Check sheet for the modelled part. Datum: model origin and axes. Units: mm. Face numbers are marked on the shaded views. A direction names the side the tool comes from. Give positions to 0.01 mm unless a question says otherwise; leave off trailing zeros. Loops run counter-clockwise (first coordinate to the right, second up) from the corner with the lowest first, then second, coordinate; pieces in that order, holes last. Notation, with made-up numbers: M 3,60.25 L 48,60.25 A18 cw 48,75.25 Z; hole C -12.75,65.25 d3. An arc over 180 degrees is marked long. One line per question, with ' | ' between items. Start each with the question number.
from build123d import *

# Parameters (mm, degrees)
F0_W         = 25.4
F0_H         = 25.4
F0_R         = 11.45
F1_DEPTH     = 7.62
F2_T1_DEPTH  = 25.4
F2_T3_DEPTH  = 25.4
F2_T5_DEPTH  = 25.4
F2_T7_DEPTH  = 25.4
F2_T10_ANGLE = 89.4745768315
F2_T12_ANGLE = 89.4745768315
F2_T14_ANGLE = 89.4745768315
F2_T16_ANGLE = 89.4745768315
F2_T18_ANGLE = 89.4745768315
F2_T20_ANGLE = 89.4745768315
F2_T22_ANGLE = 89.4745768315
F2_T24_ANGLE = 89.4745768315
F2_T29_DEPTH = 38.4641495789
F2_T33_DEPTH = 38.4641495789
F2_T40_DEPTH = 38.4641495789
F2_T44_DEPTH = 38.4641495789
F2_T51_DEPTH = 38.4641495789
F2_T55_DEPTH = 38.4641495789
F2_T62_DEPTH = 38.4641495789
F2_T66_DEPTH = 38.4641495789


# Not quite as in the source:
# - a fillet or chamfer that OpenCascade refuses, or shapes differently, is made with other operations: its cross-section is extruded or revolved along the edge and cut away or added


with BuildPart() as f1:
    # F0 (on Top) → F1 (new body)
    with BuildSketch(Plane.XY):
        Rectangle(F0_W, F0_H)
        Circle(F0_R, mode=Mode.SUBTRACT)
        with BuildLine():
            Line((8.4598493137, -38.1), (12.7, -38.1))
            Line((12.7, -38.1), (12.7, -12.7))
            Line((12.7, -12.7), (-12.7, -12.7))
            Line((-12.7, -12.7), (-12.7, -38.1))
            Line((-12.7, -38.1), (-8.4598493137, -38.1))
            ThreePointArc((-8.4598493137, -38.1), (0, -33.3121), (8.4598493137, -38.1))
        make_face()
        with BuildLine():
            ThreePointArc((0, -60.0970452561), (9.2970452561, -50.8), (12.7, -38.1))
            Line((12.7, -38.1), (8.4598493137, -38.1))
            ThreePointArc((8.4598493137, -38.1), (9.5093742552, -40.5442360341), (9.8679, -43.18))
            ThreePointArc((9.8679, -43.18), (-2.6357639659, -52.6893742552), (-8.4598493137, -38.1))
            Line((-8.4598493137, -38.1), (-12.7, -38.1))
            ThreePointArc((-12.7, -38.1), (-9.2970452561, -50.8), (0, -60.0970452561))
        make_face()
        with BuildLine():
            Line((38.1, -8.4598493137), (38.1, -12.7))
            ThreePointArc((38.1, -12.7), (50.8, -9.2970452561), (60.0970452561, 0))
            ThreePointArc((60.0970452561, 0), (50.8, 9.2970452561), (38.1, 12.7))
            Line((38.1, 12.7), (38.1, 8.4598493137))
            ThreePointArc((38.1, 8.4598493137), (48.0403764468, 8.5879095946), (53.0479, 0))
            ThreePointArc((53.0479, 0), (48.0403764468, -8.5879095946), (38.1, -8.4598493137))
        make_face()
        with BuildLine():
            Line((12.7, 12.7), (12.7, -12.7))
            Line((12.7, -12.7), (38.1, -12.7))
            Line((38.1, -12.7), (38.1, -8.4598493137))
            ThreePointArc((38.1, -8.4598493137), (33.3121, 0), (38.1, 8.4598493137))
            Line((38.1, 8.4598493137), (38.1, 12.7))
            Line((38.1, 12.7), (12.7, 12.7))
        make_face()
        with BuildLine():
            Line((-12.7, 12.7), (12.7, 12.7))
            Line((12.7, 12.7), (12.7, 38.1))
            Line((12.7, 38.1), (8.4598493137, 38.1))
            ThreePointArc((8.4598493137, 38.1), (0, 33.3121), (-8.4598493137, 38.1))
            Line((-8.4598493137, 38.1), (-12.7, 38.1))
            Line((-12.7, 38.1), (-12.7, 12.7))
        make_face()
        with BuildLine():
            Line((8.4598493137, 38.1), (12.7, 38.1))
            ThreePointArc((12.7, 38.1), (9.2970452561, 50.8), (0, 60.0970452561))
            ThreePointArc((0, 60.0970452561), (-9.2970452561, 50.8), (-12.7, 38.1))
            Line((-12.7, 38.1), (-8.4598493137, 38.1))
            ThreePointArc((-8.4598493137, 38.1), (-2.6357639659, 52.6893742552), (9.8679, 43.18))
            ThreePointArc((9.8679, 43.18), (9.5093742552, 40.5442360341), (8.4598493137, 38.1))
        make_face()
        with BuildLine():
            ThreePointArc((-60.0970452561, 0), (-50.8, -9.2970452561), (-38.1, -12.7))
            Line((-38.1, -12.7), (-38.1, -8.4598493137))
            ThreePointArc((-38.1, -8.4598493137), (-53.0479, 0), (-38.1, 8.4598493137))
            Line((-38.1, 8.4598493137), (-38.1, 12.7))
            ThreePointArc((-38.1, 12.7), (-50.8, 9.2970452561), (-60.0970452561, 0))
        make_face()
        with BuildLine():
            Line((-38.1, -12.7), (-12.7, -12.7))
            Line((-12.7, -12.7), (-12.7, 12.7))
            Line((-12.7, 12.7), (-38.1, 12.7))
            Line((-38.1, 12.7), (-38.1, 8.4598493137))
            ThreePointArc((-38.1, 8.4598493137), (-34.5920904054, 4.8603764468), (-33.3121, 0))
            ThreePointArc((-33.3121, 0), (-34.5920904054, -4.8603764468), (-38.1, -8.4598493137))
            Line((-38.1, -8.4598493137), (-38.1, -12.7))
        make_face()
    extrude(amount=F1_DEPTH)

    # F2: chamfer of 5.08 on 8 edges, made by hand

    # F2_s2 → F2_t1 (cut)
    with BuildSketch(Plane.YZ.offset(-38.1)):
        Polygon((-12.7, 2.54), (-7.62, 7.62), (-12.7, 7.62), align=None)
        Polygon((12.7, 2.54), (7.62, 7.62), (12.7, 7.62), align=None)
    extrude(amount=F2_T1_DEPTH, mode=Mode.SUBTRACT)

    # F2_s4 → F2_t3 (cut)
    with BuildSketch(Plane.XZ.offset(12.7)):
        Polygon((-12.7, 2.54), (-7.62, 7.62), (-12.7, 7.62), align=None)
        Polygon((12.7, 2.54), (7.62, 7.62), (12.7, 7.62), align=None)
    extrude(amount=F2_T3_DEPTH, mode=Mode.SUBTRACT)

    # F2_s6 → F2_t5 (cut)
    with BuildSketch(Plane.YZ.offset(12.7)):
        Polygon((-12.7, 2.54), (-7.62, 7.62), (-12.7, 7.62), align=None)
        Polygon((12.7, 2.54), (7.62, 7.62), (12.7, 7.62), align=None)
    extrude(amount=F2_T5_DEPTH, mode=Mode.SUBTRACT)

    # F2_s8 → F2_t7 (cut)
    with BuildSketch(Plane.XZ.offset(-38.1)):
        Polygon((12.7, 2.54), (7.62, 7.62), (12.7, 7.62), align=None)
        Polygon((-12.7, 2.54), (-7.62, 7.62), (-12.7, 7.62), align=None)
    extrude(amount=F2_T7_DEPTH, mode=Mode.SUBTRACT)

    # F2_s9 → F2_t10 (revolve, cut)
    with BuildSketch(Plane.YZ.offset(-38.1)):
        Polygon((12.7, 2.54), (7.62, 7.62), (12.7, 7.62), align=None)
    revolve(axis=Axis((-38.1, -12.7, 7.62), (0, 0, 1)), revolution_arc=F2_T10_ANGLE, mode=Mode.SUBTRACT)

    # F2_s11 → F2_t12 (revolve, cut)
    with BuildSketch(Plane(origin=(13.0483033064, 0.1196610486, 0), x_dir=(0, 0, 1), z_dir=(0.9999579525, 0.0091702357, 0))):
        Polygon((2.54, -63.3819359967), (7.62, -58.3019359967), (7.62, -63.3819359967), align=None)
    revolve(axis=Axis((12.7, 38.1, 7.62), (0, 0, 1)), revolution_arc=F2_T12_ANGLE, mode=Mode.SUBTRACT)

    # F2_s13 → F2_t14 (revolve, cut)
    with BuildSketch(Plane.XZ.offset(-38.1)):
        Polygon((12.7, 2.54), (7.62, 7.62), (12.7, 7.62), align=None)
    revolve(axis=Axis((-12.7, 38.1, 7.62), (0, 0, 1)), revolution_arc=F2_T14_ANGLE, mode=Mode.SUBTRACT)

    # F2_s15 → F2_t16 (revolve, cut)
    with BuildSketch(Plane(origin=(0.1196610486, -13.0483033064, 0), x_dir=(0, 0, 1), z_dir=(0.0091702357, -0.9999579525, 0))):
        Polygon((2.54, -63.3819359967), (7.62, -58.3019359967), (7.62, -63.3819359967), align=None)
    revolve(axis=Axis((38.1, -12.7, 7.62), (0, 0, 1)), revolution_arc=F2_T16_ANGLE, mode=Mode.SUBTRACT)

    # F2_s17 → F2_t18 (revolve, cut)
    with BuildSketch(Plane.YZ.offset(38.1)):
        Polygon((-12.7, 2.54), (-7.62, 7.62), (-12.7, 7.62), align=None)
    revolve(axis=Axis((38.1, 12.7, 7.62), (0, 0, 1)), revolution_arc=F2_T18_ANGLE, mode=Mode.SUBTRACT)

    # F2_s19 → F2_t20 (revolve, cut)
    with BuildSketch(Plane(origin=(-13.0483033064, -0.1196610486, 0), x_dir=(0, 0, 1), z_dir=(-0.9999579525, -0.0091702357, 0))):
        Polygon((2.54, -63.3819359967), (7.62, -58.3019359967), (7.62, -63.3819359967), align=None)
    revolve(axis=Axis((-12.7, -38.1, 7.62), (0, 0, 1)), revolution_arc=F2_T20_ANGLE, mode=Mode.SUBTRACT)

    # F2_s21 → F2_t22 (revolve, cut)
    with BuildSketch(Plane.XZ.offset(38.1)):
        Polygon((-12.7, 2.54), (-7.62, 7.62), (-12.7, 7.62), align=None)
    revolve(axis=Axis((12.7, -38.1, 7.62), (0, 0, 1)), revolution_arc=F2_T22_ANGLE, mode=Mode.SUBTRACT)

    # F2_s23 → F2_t24 (revolve, cut)
    with BuildSketch(Plane(origin=(-0.1196610486, 13.0483033064, 0), x_dir=(0, 0, 1), z_dir=(-0.0091702357, 0.9999579525, 0))):
        Polygon((2.54, -63.3819359967), (7.62, -58.3019359967), (7.62, -63.3819359967), align=None)
    revolve(axis=Axis((-38.1, 12.7, 7.62), (0, 0, 1)), revolution_arc=F2_T24_ANGLE, mode=Mode.SUBTRACT)


with BuildPart() as f2_tool27:
    # F2_s28 → F2_t29 (new body)
    with BuildSketch(Plane.YZ.offset(-38.1)):
        Polygon((-12.7, 2.54), (-7.62, 7.62), (-12.7, 7.62), align=None)
    extrude(amount=F2_T29_DEPTH)

    split(bisect_by=Plane.YZ.offset(-12.7), keep=Keep.TOP)


with BuildPart() as f2_tool31:
    # F2_s32 → F2_t33 (new body)
    with BuildSketch(Plane.XZ.offset(-0.3641495789)):
        Polygon((-12.7, 2.54), (-7.62, 7.62), (-12.7, 7.62), align=None)
    extrude(amount=F2_T33_DEPTH)

    split(bisect_by=Plane.XZ.offset(12.7), keep=Keep.BOTTOM)


with BuildPart() as f2_tool27_1:
    add(f2_tool27.part)

    # F2_t35: intersect F2_tool31
    add(f2_tool31.part, mode=Mode.INTERSECT)


with BuildPart() as f1_1:
    add(f1.part)

    # F2_t25: cut F2_tool27
    add(f2_tool27_1.part, mode=Mode.SUBTRACT)


with BuildPart() as f2_tool38:
    # F2_s39 → F2_t40 (new body)
    with BuildSketch(Plane.XZ.offset(38.1)):
        Polygon((12.7, 2.54), (7.62, 7.62), (12.7, 7.62), align=None)
    extrude(amount=-F2_T40_DEPTH)

    split(bisect_by=Plane.XZ.offset(12.7), keep=Keep.BOTTOM)


with BuildPart() as f2_tool42:
    # F2_s43 → F2_t44 (new body)
    with BuildSketch(Plane.YZ.offset(-0.3641495789)):
        Polygon((-12.7, 2.54), (-7.62, 7.62), (-12.7, 7.62), align=None)
    extrude(amount=F2_T44_DEPTH)

    split(bisect_by=Plane.YZ.offset(12.7), keep=Keep.BOTTOM)


with BuildPart() as f2_tool38_1:
    add(f2_tool38.part)

    # F2_t46: intersect F2_tool42
    add(f2_tool42.part, mode=Mode.INTERSECT)


with BuildPart() as f1_2:
    add(f1_1.part)

    # F2_t36: cut F2_tool38
    add(f2_tool38_1.part, mode=Mode.SUBTRACT)


with BuildPart() as f2_tool49:
    # F2_s50 → F2_t51 (new body)
    with BuildSketch(Plane.YZ.offset(38.1)):
        Polygon((12.7, 2.54), (7.62, 7.62), (12.7, 7.62), align=None)
    extrude(amount=-F2_T51_DEPTH)

    split(bisect_by=Plane.YZ.offset(12.7), keep=Keep.BOTTOM)


with BuildPart() as f2_tool53:
    # F2_s54 → F2_t55 (new body)
    with BuildSketch(Plane.XZ.offset(0.3641495789)):
        Polygon((12.7, 2.54), (7.62, 7.62), (12.7, 7.62), align=None)
    extrude(amount=-F2_T55_DEPTH)

    split(bisect_by=Plane.XZ.offset(-12.7), keep=Keep.TOP)


with BuildPart() as f2_tool49_1:
    add(f2_tool49.part)

    # F2_t57: intersect F2_tool53
    add(f2_tool53.part, mode=Mode.INTERSECT)


with BuildPart() as f1_3:
    add(f1_2.part)

    # F2_t47: cut F2_tool49
    add(f2_tool49_1.part, mode=Mode.SUBTRACT)


with BuildPart() as f2_tool60:
    # F2_s61 → F2_t62 (new body)
    with BuildSketch(Plane.XZ.offset(-38.1)):
        Polygon((-12.7, 2.54), (-7.62, 7.62), (-12.7, 7.62), align=None)
    extrude(amount=F2_T62_DEPTH)

    split(bisect_by=Plane.XZ.offset(-12.7), keep=Keep.TOP)


with BuildPart() as f2_tool64:
    # F2_s65 → F2_t66 (new body)
    with BuildSketch(Plane.YZ.offset(0.3641495789)):
        Polygon((12.7, 2.54), (7.62, 7.62), (12.7, 7.62), align=None)
    extrude(amount=-F2_T66_DEPTH)

    split(bisect_by=Plane.YZ.offset(-12.7), keep=Keep.TOP)


with BuildPart() as f2_tool60_1:
    add(f2_tool60.part)

    # F2_t68: intersect F2_tool64
    add(f2_tool64.part, mode=Mode.INTERSECT)


with BuildPart() as f1_4:
    add(f1_3.part)

    # F2_t58: cut F2_tool60
    add(f2_tool60_1.part, mode=Mode.SUBTRACT)


solid = f1_4.part
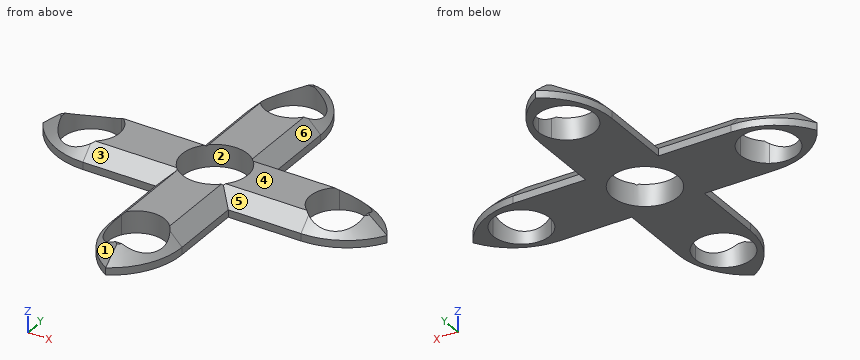
Q1. Cross-section at B-B (x = 4). State how many separate pieces and enclosed holes the cut face has, and give its area (3 significant figures).
Q2. Cross-section at A-A (y = -29). Record the cut outline in (x, z).
Q3. Draft check along X on the marked faces 1, 2 and 3. Enter one of: released by +X, released by -X, zero draft, split by the parting line, or undercut.
Q4. Material ranges on probe 1 along X at (y, z) = (-43.18, 2); probe 2 along X at (y, z) = (13, 6.75); probe 3 along X at (y, z) = (-41, 4.5), recorded low to high. Write a range as from..to.
Q5. Access from +Z, -Z, +X, -X, +Y, -Y to the whole of each face (thin tool, end or side, straight path). Record for the marked faces 4, 5 and 6.
Q6. Depth check by flat-ended pin: P1, Ø0.8, axis at y = 30.5, z = 1.5, coming from the +X side; P2, Ø2, axis at x = -24, z = 1, coming from the -Y side; P3, Ø1.5, axis at x = -20, y = 2.5, coming from the -Z side; P4, Ø1.3, axis at y = 27.5, z = 1, coming from the -X side. Enter the tip coordinate at first touch or a pass-through.
Solved:
1) separate pieces: 4 | enclosed holes: 0 | area: 401 mm²
2) outline: M -12.7,0 L 12.7,0 L 12.7,2.54 L 7.62,7.62 L -7.62,7.62 L -12.7,2.54 Z
3) face 1: released by -X | face 2: undercut | face 3: zero draft
4) probe 1: x = -12.19..-9.87, 9.87..12.19 | probe 2: x = -8.49..8.49 | probe 3: x = -10.56..-9.62, 9.62..10.56
5) face 4: +Z, +X, -X, +Y, -Y | face 5: +Z, +X, -Y | face 6: +Z, +X, +Y
6) P1: stops at x = 12.7 | P2: stops at y = -12.7 | P3: stops at z = 0 | P4: stops at x = -12.7
